Here's how the part is built. I have some questions about the finished solid (model axes, mm). Face numbers are marked on the shaded views. A direction names the side the tool comes from. Give positions to 0.01 mm unless a question says otherwise; leave off trailing zeros. Loops run counter-clockwise (first coordinate to the right, second up) from the corner with the lowest first, then second, coordinate; pieces in that order, holes last. Notation, with made-up numbers: (62, 68.25) -> (92, 68.25) arc R20 cw to (92, 82.25) -> close; hole circle Ø3 at (-18.75, 44.5). An arc over 180 degrees is marked (long way). Answer in a Markdown table with one row per item. Add a question column.
Item 1: If we section it at A-A (y = 7): Give the number of separate pieces and of enclosed holes in the cut face, then the cut area to 3 significant figures.
Item 2: If we section it at C-C (x = -4): Write out the boundary of the cut face in (y, z).
Item 3: We'd pull the mould along Z, two halves only. Please class the marked faces 1, 2, 3 and 4: released by +Z, released by -Z, zero draft, split by the parting line, or undercut.
Item 4: For P1, Ø4, axis at x = -23, y = -3.5, coming from the -Z side; P2, Ø1.6, axis at y = 4.5, z = 22.5, coming from the +X side; P3, Ø2.5, axis at x = -34.81, y = 7, coming from the -Z side; P4, Ø10, axis at x = -37.5, z = 18, coming from the -Y side, each with a flat end and sliding along its axis, tell me the tip position at first contact or that it passes through.
Item 5: If we section it at B-B (z = -1.5): Write out the boundary of the cut face in (x, y), then the cut area to 3 significant figures.
Item 6: If we section it at D-D (x = -20): Write out the boundary of the cut face in (y, z).
Item 7: If I drill on line 1 (Z direction, x = 0.5, y = 8); line 2 (X direction, y = -15.25, z = 3.5); line 3 (Y direction, x = 3, z = -11), over which ranges is the centre line in solid material (lowest first)?
Item 8: Which directions (+Z, -Z, +X, -X, +Y, -Y) give clear straight access to the entire face, cutting with the end or side of a thin tool? Please do the marked faces 5, 6 and 7.
```python
from build123d import *

# Parameters (mm, degrees)
SKETCH1_W           = 55
SKETCH1_H           = 40
BOSS_EXTRUDE1_DEPTH = 2
SKETCH3_W           = 15
SKETCH3_H           = 2
BOSS_EXTRUDE2_DEPTH = 10
FILLET1_R           = 3
FILLET2_R           = 3
FILLET3_R           = 3
FILLET4_R           = 3
SKETCH4_R           = 1.5
CUT_EXTRUDE1_DEPTH  = 50
SKETCH5_W           = 53.242640687
SKETCH5_H           = 38.242640688
BOSS_EXTRUDE3_DEPTH = 13
CUT_EXTRUDE2_DEPTH  = 61.469324671
SKETCH7_R           = 0.75
BOSS_EXTRUDE4_DEPTH = 4


with BuildPart() as part:
    # Sketch1 → Boss-Extrude1 (new body)
    with BuildSketch(Plane(origin=(0, 0, 0), x_dir=(1, 0, 0), z_dir=(0, 1, 0))):
        with Locations((-17.80952381, -3.630952381)):
            Rectangle(SKETCH1_W, SKETCH1_H)
    extrude(amount=BOSS_EXTRUDE1_DEPTH)

    # Sketch3 → Boss-Extrude2 (add)
    with BuildSketch(Plane(origin=(0, 2, 0), x_dir=(1, 0, 0), z_dir=(0, 1, 0))):
        with Locations((-34.80952381, 15.369047619)):
            Rectangle(SKETCH3_W, SKETCH3_H)
        with Locations((-34.80952381, -22.630952381)):
            Rectangle(SKETCH3_W, SKETCH3_H)
        with Locations((-0.80952381, -22.630952381)):
            Rectangle(SKETCH3_W, SKETCH3_H)
        with Locations((-0.80952381, 15.369047619)):
            Rectangle(SKETCH3_W, SKETCH3_H)
    extrude(amount=BOSS_EXTRUDE2_DEPTH)

    # Fillet1
    fillet1_edges = [part.edges().sort_by_distance(p)[0] for p in [
        (-45.30952381, 1, -16.369047619),
    ]]
    fillet(fillet1_edges, radius=FILLET1_R)

    # Fillet2
    fillet2_edges = [part.edges().sort_by_distance(p)[0] for p in [
        (-45.30952381, 1, 23.630952381),
    ]]
    fillet(fillet2_edges, radius=FILLET2_R)

    # Fillet3
    fillet3_edges = [part.edges().sort_by_distance(p)[0] for p in [
        (9.69047619, 1, -16.369047619),
    ]]
    fillet(fillet3_edges, radius=FILLET3_R)

    # Fillet4
    fillet4_edges = [part.edges().sort_by_distance(p)[0] for p in [
        (9.69047619, 1, 23.630952381),
    ]]
    fillet(fillet4_edges, radius=FILLET4_R)

    # Sketch4 → Cut-Extrude1 (cut)
    with BuildSketch(Plane.XY.offset(23.630952381)):
        with Locations((-0.80952381, 7)):
            Circle(SKETCH4_R)
        with Locations((-34.80952381, 7)):
            Circle(SKETCH4_R)
    extrude(amount=-CUT_EXTRUDE1_DEPTH, mode=Mode.SUBTRACT)

    # Sketch5 → Boss-Extrude3 (add)
    with BuildSketch(Plane.XZ):
        with Locations((-17.809523809, 3.630952381)):
            Rectangle(SKETCH5_W, SKETCH5_H)
    extrude(amount=BOSS_EXTRUDE3_DEPTH)

    # Sketch6 → Cut-Extrude2 (cut, through all)
    with BuildSketch(Plane.ZY.offset(44.430844153)):
        Polygon((-15.490367963, -13), (-12.490367963, -13), (-15.490367963, 0), align=None)
        Polygon((19.752272725, -13), (22.752272725, 0), (22.752272725, -13), align=None)
    extrude(amount=-CUT_EXTRUDE2_DEPTH, mode=Mode.SUBTRACT)

    # Sketch7 → Boss-Extrude4 (add)
    with BuildSketch(Plane.XZ.offset(13)):
        with Locations(Location((-17.80952381, 3.630952381, 0), (0, 0, 90))):
            Circle(SKETCH7_R)
    extrude(amount=BOSS_EXTRUDE4_DEPTH)


solid = part.part
```
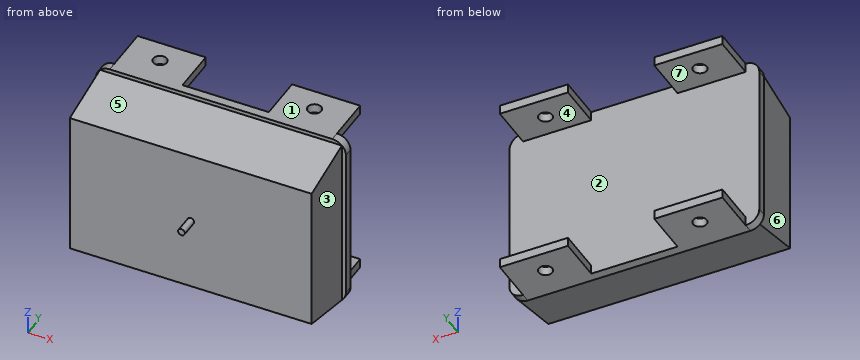
Recorded:
| question | item | result |
|---|---|---|
| 1 | separate pieces | 8 |
| 1 | enclosed holes | 0 |
| 1 | area | 96.0 mm^2 |
| 2 | outline | (-13, -12.49) -> (0, -15.49) -> (0, -16.37) -> (12, -16.37) -> (12, -14.37) -> (2, -14.37) -> (2, 21.63) -> (12, 21.63) -> (12, 23.63) -> (0, 23.63) -> (0, 22.75) -> (-13, 19.75) -> close |
| 3 | face 1 | released by +Z |
| 3 | face 2 | undercut |
| 3 | face 3 | zero draft |
| 3 | face 4 | undercut |
| 4 | P1 | stops at z = -15.14 |
| 4 | P2 | stops at x = 6.69 |
| 4 | P3 | passes through |
| 4 | P4 | stops at y = -13 |
| 5 | outline | (-45.31, 0) -> (-44.43, 0) -> (-44.43, -13) -> (8.81, -13) -> (8.81, 0) -> (9.69, 0) -> (9.69, 2) -> (-45.31, 2) -> close |
| 5 | area | 802 mm^2 |
| 6 | outline | (-13, -12.49) -> (0, -15.49) -> (0, -16.37) -> (2, -16.37) -> (2, 23.63) -> (0, 23.63) -> (0, 22.75) -> (-13, 19.75) -> close |
| 7 | line 1 | z = -16.37 to -14.37, 21.63 to 23.63 |
| 7 | line 2 | x = -18.55 to -17.07 |
| 7 | line 3 | y = -13 to 2 |
| 8 | face 5 | +Z, +X, -X, -Y |
| 8 | face 6 | +Z, -Z, -X, -Y |
| 8 | face 7 | +X, -X, +Y |
